Build history of the part. All positions in model axes, mm. A direction names the side the tool comes from. Give positions to 0.01 mm unless a question says otherwise; leave off trailing zeros. Loops run counter-clockwise (first coordinate to the right, second up) from the corner with the lowest first, then second, coordinate; pieces in that order, holes last. Notation, with made-up numbers: M 80.5,86.25 L 139.5,86.25 A20 ccw 139.5,101.25 Z; hole C 17,-15.75 d4. An arc over 180 degrees is marked long. Answer as a JSON object with one key per item and string values. Group by question number.
1. Drill centre lines: line 1 along Y through (x, z) = (27.5, 0); line 2 along Y through (x, z) = (31, -1.5); line 3 along X through (y, z) = (0, -1.25). Where is each one in solid material? Low to high. Write a range as [from, to].
2. 3-axis set-ups, long thin cutter, end or side, ignore diameter. For faces 1 (the face through (-22.5, 0, 0)), 2 (the face through (37.5, -1, 2)), 3 (the face through (22.5, 0, 0)): which of +Z, -Z, +X, -X, +Y, -Y reach the whole face in a straight line?
3. Slice it at D-D (z = -2.75). List the corners of the cut face in (x, y), then the cut area to 3 significant figures.
4. Drop flat-ended pins along their axis: pin 1 Ø2 at (y, z) = (0, 0.5) entering from +X; pin 2 Ø1 at (x, y) = (-20, -1.5) entering from -Z; pin 3 Ø3 at (x, z) = (-4.5, 2.5) entering from +Y. Give the stop position or say it passes through.
5. Slice it at A-A (x = 24.5). List the corners of the cut face in (y, z).
6. Mould opens along Y. For faces 4 (the face through (-37.5, -1, 2)), 5 (the face through (-30, 2, 0)), 6 (the face through (30, -2, 0)), 7 (the face through (0.525, -3.905, 0.867)) say: released by +Y, released by -Y, zero draft, split by the parting line, or undercut.
7. Slice it at B-B (z = 0). List the corners of the cut face in (x, y), then the cut area to 3 significant figures.
from build123d import *

# Parameters (mm, degrees)
SKETCH1_R           = 4
BOSS_EXTRUDE1_DEPTH = 37.5
SKETCH2_R           = 2
CUT_EXTRUDE1_DEPTH  = 15
CUT_EXTRUDE2_START  = -15
SKETCH3_R           = 2
CUT_EXTRUDE2_DEPTH  = 15


with BuildPart() as part:
    # Sketch1 → Boss-Extrude1 (new, symmetric)
    with BuildSketch(Plane(origin=(0, 0, 0), x_dir=(0, 0, -1), z_dir=(1, 0, 0))):
        Circle(SKETCH1_R)
    extrude(amount=BOSS_EXTRUDE1_DEPTH, both=True)

    # Sketch2 → Cut-Extrude1 (cut)
    with BuildSketch(Plane(origin=(37.5, 0, 0), x_dir=(0, 0, -1), z_dir=(1, 0, 0))):
        Circle(SKETCH2_R)
    extrude(amount=-CUT_EXTRUDE1_DEPTH, mode=Mode.SUBTRACT)

    # Sketch3 → Cut-Extrude2 (cut)
    with BuildSketch(Plane.ZY.offset(37.5).offset(CUT_EXTRUDE2_START)):
        with Locations(Location((0, 0, 0), (0, 0, 180))):
            Circle(SKETCH3_R)
    extrude(amount=CUT_EXTRUDE2_DEPTH, mode=Mode.SUBTRACT)


solid = part.part
Established:
{
 "1": {"line 1": "y = [-4, -2], [2, 4]", "line 2": "y = [-3.71, -1.32], [1.32, 3.71]", "line 3": "x = [-22.5, 22.5]"},
 "2": {"face 1": "-X", "face 2": "+Z, -Z, +X, +Y, -Y", "face 3": "+X"},
 "3": {"outline": "M -37.5,-2.9 L 37.5,-2.9 L 37.5,2.9 L -37.5,2.9 Z", "area": "436 mm^2"},
 "4": {"pin 1": "stops at x = 22.5", "pin 2": "stops at z = -3.87", "pin 3": "stops at y = 3.87"},
 "5": {"outline": "C 0,0 d8; hole C 0,0 d4"},
 "6": {"face 4": "zero draft", "face 5": "undercut", "face 6": "undercut", "face 7": "split by the parting line"},
 "7": {"outline": "M -37.5,-4 L 37.5,-4 L 37.5,-2 L 22.5,-2 L 22.5,2 L 37.5,2 L 37.5,4 L -37.5,4 L -37.5,2 L -22.5,2 L -22.5,-2 L -37.5,-2 Z", "area": "480 mm^2"}
}
